Model file for the job. Use its own axes, mm. A direction names the side the tool comes from. Give positions to 0.01 mm unless a question says otherwise; leave off trailing zeros. Order: outer loops, then holes, each group sorted by start corner. A loop starts at its lowest first (then second) coordinate and runs counter-clockwise, first axis right, second up. Notation, with made-up numbers: (68.5, -35) - (90.5, -35) arc R29 cw to (90.5, -8) - close; hole circle Ø5 at (27.25, 5.5). An arc over 180 degrees is marked (long way). Use CSV: the item, a comma, the result in double quotes. Start each with the question number.
(1) Drop flat-ended pins along their axis: pin 1 Ø1.2 at (x, z) = (1.5, 0.5) entering from +Y; pin 2 Ø6 at (x, y) = (1, -2) entering from -Z; pin 3 Ø1 at (x, z) = (-2, 3) entering from +Y; pin 4 Ø1.2 at (y, z) = (-1.5, 0.5) entering from -X. Give the stop position or say it passes through.
(2) Probe L1, parallel to X at y = -2.75, z = 3.05; L2, parallel to Y at x = 3, z = 0.4; L3, parallel to X at y = -4.5, z = 3.15. List the from-to ranges inside material, lowest first.
(3) Tool access for faces 4 (the flat face through (5.15, 0, 1)), 5 (the flat face through (0, 7, 3.5)), 6 (the cylindrical face through (5.64, 5.65, 2.51)): list every direction of +Z, -Z, +X, -X, +Y, -Y with a clear straight run to the whole face (end or side of a thin tool).
(4) Band-saw the part on A-A, the plane z = 1.2. Give the cut face in (x, y).
(5) Band-saw the part on C-C, the plane x = 3. Give the cut face in (y, z).
(6) Band-saw the part on D-D, the plane z = 2.75. Give the cut face in (x, y).
(7) Band-saw the part on B-B, the plane y = 0.75. Give the cut face in (x, z), then the cut area to 3 significant figures.
(8) Pull direction X, two halves, no side cores. Call faces 1 (the flat face through (8.335, 3.396, 1.726)), 2 (the flat face through (6.15, 0, 2)), 3 (the flat face through (-8.295, 3.492, 1.726)): +X half, -X half, draft (parallel to the pull), parting line (faces both ways), or undercut.
from build123d import *

# Parameters (mm, degrees)
BOSS_EXTRUDE1_DEPTH = 1.5
SKETCH2_W           = 12.3
SKETCH2_H           = 10.3
BOSS_EXTRUDE2_DEPTH = 2
CUT_EXTRUDE1_DEPTH  = 2
CUT_EXTRUDE2_REACH  = 5.5


with BuildPart() as part:
    # Sketch1 → Boss-Extrude1 (new body)
    with BuildSketch(Plane.XY):
        Polygon((6.888301783, 6.888301783), (0, 9.741529803), (-6.888301783, 6.888301783), (-9.741529803, 0), (-6.888301783, -6.888301783), (0, -9.741529803), (6.888301783, -6.888301783), (9.741529803, 0), align=None)
        with BuildLine():
            Line((-5.15, -3.65), (-5.15, 3.65))
            ThreePointArc((-5.15, 3.65), (-5.003553391, 4.003553391), (-4.65, 4.15))
            Line((-4.65, 4.15), (4.65, 4.15))
            ThreePointArc((4.65, 4.15), (5.003553391, 4.003553391), (5.15, 3.65))
            Line((5.15, 3.65), (5.15, -3.65))
            ThreePointArc((5.15, -3.65), (5.003553391, -4.003553391), (4.65, -4.15))
            Line((4.65, -4.15), (-4.65, -4.15))
            ThreePointArc((-4.65, -4.15), (-5.003553391, -4.003553391), (-5.15, -3.65))
        make_face(mode=Mode.SUBTRACT)
    extrude(amount=BOSS_EXTRUDE1_DEPTH)

    # Sketch2 → Boss-Extrude2 (add)
    with BuildSketch(Plane.XY.offset(1.5)):
        Polygon((9.741529803, 0), (6.888301783, 6.888301783), (0, 9.741529803), (-6.888301783, 6.888301783), (-9.741529803, 0), (-6.888301783, -6.888301783), (0, -9.741529803), (6.888301783, -6.888301783), align=None)
        Rectangle(SKETCH2_W, SKETCH2_H, mode=Mode.SUBTRACT)
    extrude(amount=BOSS_EXTRUDE2_DEPTH)

    # Sketch3 → Cut-Extrude1 (cut)
    with BuildSketch(Plane.XY.offset(3.5)):
        with BuildLine():
            Line((-6.15, -5.15), (-6.15, 5.15))
            ThreePointArc((-6.15, 5.15), (-5.65, 5.65), (-5.15, 5.15))
            Line((-5.15, 5.15), (-5.15, -5.15))
            ThreePointArc((-5.15, -5.15), (-5.65, -5.65), (-6.15, -5.15))
        make_face()
        with BuildLine():
            Line((5.15, -5.15), (5.15, 5.15))
            ThreePointArc((5.15, 5.15), (5.65, 5.65), (6.15, 5.15))
            Line((6.15, 5.15), (6.15, -5.15))
            ThreePointArc((6.15, -5.15), (5.65, -5.65), (5.15, -5.15))
        make_face()
    extrude(amount=-CUT_EXTRUDE1_DEPTH, mode=Mode.SUBTRACT)

    # Sketch4 → Cut-Extrude2 (cut, up to next)
    with BuildSketch(Plane.XY.offset(3.5), mode=Mode.PRIVATE) as cut_extrude2_sk1:
        Polygon((-6.888301783, -6.888301783), (6.888301783, -6.888301783), (0, -9.741529803), align=None)
    cut_extrude2_tool1 = extrude(cut_extrude2_sk1.sketch, amount=-CUT_EXTRUDE2_REACH, mode=Mode.PRIVATE) & part.part
    add(cut_extrude2_tool1.solids().sort_by_distance((0, -7.839378, 3.5))[0], mode=Mode.SUBTRACT)


solid = part.part
Answer block:
1,pin 1,"stops at y = 9.37"
1,pin 2,"stops at z = 0"
1,pin 3,"stops at y = 9.12"
1,pin 4,"stops at x = -9.37"
2,L1,"x = -8.6 to -6.15, 6.15 to 8.6"
2,L2,"y = -6.89 to -4.15, 4.15 to 8.5"
2,L3,"x = -7.88 to -6.15, 6.15 to 7.88"
3,face 4,"+Z, -Z"
3,face 5,"+Z, +X, -X, +Y, -Y"
3,face 6,"+Z"
4,outline,"(-9.74, 0) - (-6.89, -6.89) - (6.89, -6.89) - (9.74, 0) - (6.89, 6.89) - (0, 9.74) - (-6.89, 6.89) - close; hole (-5.15, -3.65) arc R0.5 ccw to (-4.65, -4.15) - (4.65, -4.15) arc R0.5 ccw to (5.15, -3.65) - (5.15, 3.65) arc R0.5 ccw to (4.65, 4.15) - (-4.65, 4.15) arc R0.5 ccw to (-5.15, 3.65) - close"
5,outline,"(-6.89, 0) - (-4.15, 0) - (-4.15, 1.5) - (-5.15, 1.5) - (-5.15, 3.5) - (-6.89, 3.5) - close; (4.15, 0) - (8.5, 0) - (8.5, 3.5) - (5.15, 3.5) - (5.15, 1.5) - (4.15, 1.5) - close"
6,outline,"(-9.74, 0) - (-6.89, -6.89) - (6.89, -6.89) - (9.74, 0) - (6.89, 6.89) - (0, 9.74) - (-6.89, 6.89) - close; hole (-6.15, -5.15) arc R0.5 ccw to (-5.15, -5.15) - (5.15, -5.15) arc R0.5 ccw to (6.15, -5.15) - (6.15, 5.15) arc R0.5 ccw to (5.15, 5.15) - (-5.15, 5.15) arc R0.5 ccw to (-6.15, 5.15) - close"
7,outline,"(-9.43, 0) - (-5.15, 0) - (-5.15, 1.5) - (-6.15, 1.5) - (-6.15, 3.5) - (-9.43, 3.5) - close; (5.15, 0) - (9.43, 0) - (9.43, 3.5) - (6.15, 3.5) - (6.15, 1.5) - (5.15, 1.5) - close"
7,area,"26.0 mm2"
8,face 1,"+X half"
8,face 2,"undercut"
8,face 3,"-X half"
